from build123d import *
from build123d.topology import SkipClean

# Parameters (mm, degrees)
SKETCH1_R           = 21.1
BOSS_EXTRUDE1_DEPTH = 27.6
SKETCH2_R           = 38.25
BOSS_EXTRUDE2_DEPTH = 27.3
SKETCH3_R           = 42.5
BOSS_EXTRUDE3_DEPTH = 1.5
SKETCH4_R           = 2.1
BOSS_EXTRUDE4_DEPTH = 1
CIRPATTERN1_COUNT   = 4
DRAFT1_ANGLE        = 10
FILLET1_R           = 3
FILLET2_R           = 3


with BuildPart() as part:
    # Sketch1 → Boss-Extrude1 (new body)
    with BuildSketch(Plane(origin=(0, 0, 0), x_dir=(1, 0, 0), z_dir=(0, 1, 0))):
        with Locations(Location((0, 0, 0), (0, 0, 90))):
            Circle(SKETCH1_R)
    extrude(amount=BOSS_EXTRUDE1_DEPTH)

    # Sketch2 → Boss-Extrude2 (add)
    with BuildSketch(Plane(origin=(0, 27.6, 0), x_dir=(1, 0, 0), z_dir=(0, 1, 0))):
        with Locations(Location((0, 0, 0), (0, 0, 270))):
            Circle(SKETCH2_R)
    extrude(amount=BOSS_EXTRUDE2_DEPTH)

    # Sketch3 → Boss-Extrude3 (add)
    with BuildSketch(Plane(origin=(0, 54.9, 0), x_dir=(1, 0, 0), z_dir=(0, 1, 0))):
        with Locations(Location((0, 0, 0), (0, 0, 270))):
            Circle(SKETCH3_R)
    extrude(amount=BOSS_EXTRUDE3_DEPTH)

    # Sketch4 → Boss-Extrude4 (add)
    with BuildSketch(Plane(origin=(0, 56.4, 0), x_dir=(1, 0, 0), z_dir=(0, 1, 0))):
        with BuildLine():
            Line((-23.216565266, 37.376344086), (-2.374421448, 50.322580645))
            ThreePointArc((-2.374421448, 50.322580645), (0, 51), (2.374421448, 50.322580645))
            Line((2.374421448, 50.322580645), (23.216565266, 37.376344086))
            ThreePointArc((23.216565266, 37.376344086), (0, -44), (-23.216565266, 37.376344086))
        make_face()
        with Locations(Location((0, 46.5, 0), (0, 0, 270))):
            Circle(SKETCH4_R, mode=Mode.SUBTRACT)
    boss_extrude4 = extrude(amount=BOSS_EXTRUDE4_DEPTH)

    # CirPattern1: Boss-Extrude4 ×4 about axis
    cirpattern1_axis = Axis((0, 0, 0), (0, 1, 0))
    for i in range(1, CIRPATTERN1_COUNT):
        add(boss_extrude4.rotate(cirpattern1_axis, i * 360 / CIRPATTERN1_COUNT))

    # Draft1
    draft1_faces = [part.faces().sort_by_distance(p)[0] for p in [
        (0, 41.25, -38.25),
    ]]
    draft(draft1_faces, Plane(origin=(0, 54.9, 0), x_dir=(0, 0, -1), z_dir=(0, -1, 0)), DRAFT1_ANGLE)

    # Fillet1
    fillet1_edges = [part.edges().sort_by_distance(p)[0] for p in [
        (0, 0, 21.1),
    ]]
    fillet(fillet1_edges, radius=FILLET1_R)

    # Fillet2
    fillet2_edges = [part.edges().sort_by_distance(p)[0] for p in [
        (0, 27.6, -33.436273427),
    ]]
    fillet(fillet2_edges, radius=FILLET2_R)

    # Sketch6 → Cut-Revolve1 (revolve, cut)
    with BuildSketch(Plane(origin=(0, 0, 0), x_dir=(0, 0, -1), z_dir=(1, 0, 0))):
        with BuildLine():
            ThreePointArc((25.599913717, 57.391292677), (25.601491738, 57.395647071), (25.603073792, 57.4))
            Line((25.603073792, 57.4), (23.216565266, 57.4))
            Line((23.216565266, 57.4), (2.374421448, 57.4))
            Line((2.374421448, 57.4), (0, 57.4))
            Line((0, 57.4), (0, 49.4))
            ThreePointArc((0, 49.4), (13.409104565, 51.444256324), (25.599913717, 57.391292677))
        make_face()
    revolve(axis=Axis((0, 49.4, 0), (0, 1, 0)), mode=Mode.SUBTRACT)

    # Sketch6<4> → Revolve1 (revolve)
    with SkipClean():  # the faces are left unmerged after this step: merging them gives an invalid solid
        with BuildSketch(Plane(origin=(0, 0, 0), x_dir=(0, 0, -1), z_dir=(1, 0, 0))):
            with BuildLine():
                Line((25.603073792, 57.4), (35, 57.4))
                ThreePointArc((35, 57.4), (30.301536896, 60.689899283), (25.603073792, 57.4))
            make_face()
        revolve(axis=Axis((0, 49.4, 0), (0, 1, 0)))


solid = part.part
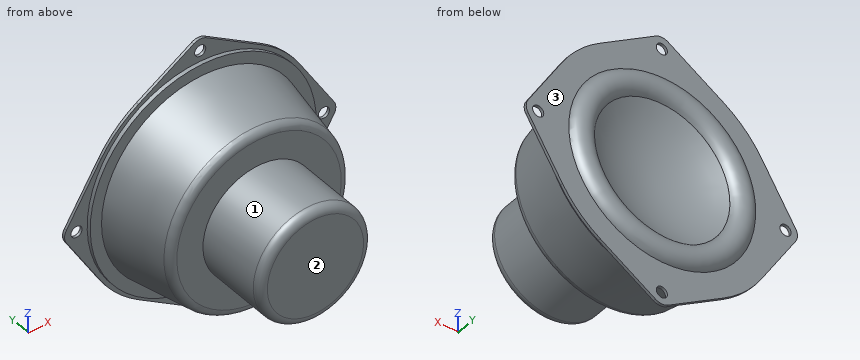
Work out the finished part from the listing and answer in its coordinate system (mm). Face numbers are marked on the shaded views. A direction names the side the tool comes from. Give positions to 0.01 mm unless a question says otherwise; leave off trailing zeros. Loops run counter-clockwise (first coordinate to the right, second up) from the corner with the lowest first, then second, coordinate; pieces in that order, holes last. Notation, with made-up numbers: (37.5, 32) - (67.5, 32) arc R25 ccw to (67.5, 64) - close; hole circle Ø7 at (-31.5, 66.5). An arc over 180 degrees is marked (long way). Answer in a Markdown table with one row per item. Add a question column.
Q1. A tool of negligible diameter and unlimited length cuts with its end or side. For the marked faces 1, 2 and 3, from which of +Z, -Z, +X, -X, +Y, -Y can it reach the whole face along a straight path? Write none if from no direction.
Q2. The part is cut by section D-D (x = 46.5). Determine the outline of the cut face in (y, z), and give its area (3 significant figures).
Q3. The part is cut by section A-A (z = 0). State how many separate pieces and enclosed holes the cut face has, and give its area (3 significant figures).
Q4. Each of these flat-tipped pins is pushed along its axis until it touches: P1, Ø4, axis at x = -37, y = 54, coming from the +Z side; P2, Ø6, axis at x = -6, y = 12.5, coming from the +Z side; P3, Ø1.5, axis at x = 3, z = -20, coming from the +Y side. Where does it stop, or does it pass through?
Q5. The part is cut by section C-C (z = 46.5). Determine the outline of the cut face in (x, y), and give its area (3 significant figures).
Q6. Consider line 1 along Y through (x, z) = (-44.5, -2); line 2 along Z through (x, y) = (46.5, 56.7). Determine where each line is inside the solid, lowest interval first.
Solution:
| question | item | result |
|---|---|---|
| 1 | face 1 | -Y |
| 1 | face 2 | +Z, -Z, +X, -X, -Y |
| 1 | face 3 | +Y |
| 2 | outline | (56.4, -8.53) - (57.4, -8.53) - (57.4, -2.1) - (56.4, -2.1) - close; (56.4, 2.1) - (57.4, 2.1) - (57.4, 8.53) - (56.4, 8.53) - close |
| 2 | area | 12.9 mm² |
| 3 | separate pieces | 3 |
| 3 | enclosed holes | 0 |
| 3 | area | 3,100 mm² |
| 4 | P1 | stops at z = 23.8 |
| 4 | P2 | stops at z = 20.89 |
| 4 | P3 | stops at y = 54.59 |
| 5 | outline | (-8.53, 56.4) - (-2.1, 56.4) - (-2.1, 57.4) - (-8.53, 57.4) - close; (2.1, 56.4) - (8.53, 56.4) - (8.53, 57.4) - (2.1, 57.4) - close |
| 5 | area | 12.9 mm² |
| 6 | line 1 | y = 56.4 to 57.4 |
| 6 | line 2 | z = -8.53 to -2.1, 2.1 to 8.53 |
